```python
from build123d import *

# Parameters (mm, degrees)
SKETCH1_W           = 61
SKETCH1_H           = 36
SKETCH1_R           = 2.5
BOSS_EXTRUDE1_DEPTH = 5
BOSS_EXTRUDE3_START = -18
BOSS_EXTRUDE3_DEPTH = 6
BOSS_EXTRUDE2_DEPTH = 12
FILLET1_R           = 1.5
FILLET2_R           = 1.5
FILLET3_R           = 1.5
FILLET4_R           = 1.5
SKETCH5_W           = 61
SKETCH5_H           = 36
SKETCH5_R           = 2.5
BOSS_EXTRUDE4_DEPTH = 5
FILLET5_R           = 1.5
FILLET6_R           = 1.5
FILLET7_R           = 1.5


with BuildPart() as part:
    # Sketch1 → Boss-Extrude1 (new body)
    with BuildSketch(Plane(origin=(0, 0, 0), x_dir=(1, 0, 0), z_dir=(0, 1, 0))):
        Rectangle(SKETCH1_W, SKETCH1_H)
        with Locations(Location((-25.5, 13.49396263, 0), (0, 0, 270))):
            Circle(SKETCH1_R, mode=Mode.SUBTRACT)
        with Locations(Location((25.5, 13.49396263, 0), (0, 0, 270))):
            Circle(SKETCH1_R, mode=Mode.SUBTRACT)
        with Locations(Location((25.5, -13, 0), (0, 0, 270))):
            Circle(SKETCH1_R, mode=Mode.SUBTRACT)
        with Locations(Location((-25.5, -13, 0), (0, 0, 270))):
            Circle(SKETCH1_R, mode=Mode.SUBTRACT)
    extrude(amount=BOSS_EXTRUDE1_DEPTH)

    # Sketch4 → Boss-Extrude3 (add, symmetric)
    with BuildSketch(Plane.XY.offset(18).offset(BOSS_EXTRUDE3_START)):
        Polygon((19.75, 5), (-17.25, 35), (-27.25, 35), (9.75, 5), align=None)
    extrude(amount=BOSS_EXTRUDE3_DEPTH, both=True)

    # Sketch3 → Boss-Extrude2 (add)
    with BuildSketch(Plane.XY.offset(18)):
        Polygon((-19.75, 5), (11.5, 35), (21.5, 35), (-9.75, 5), align=None)
    boss_extrude2 = extrude(amount=-BOSS_EXTRUDE2_DEPTH)

    # Mirror1: Boss-Extrude2 across plane
    add(boss_extrude2.mirror(Plane.XY))

    # Fillet1
    fillet1_edges = [part.edges().sort_by_distance(p)[0] for p in [
        (-9.75, 5, 12),
    ]]
    fillet(fillet1_edges, radius=FILLET1_R)

    # Fillet2
    fillet2_edges = [part.edges().sort_by_distance(p)[0] for p in [
        (-9.75, 5, -12),
    ]]
    fillet(fillet2_edges, radius=FILLET2_R)

    # Fillet3
    fillet3_edges = [part.edges().sort_by_distance(p)[0] for p in [
        (9.75, 5, 0),
    ]]
    fillet(fillet3_edges, radius=FILLET3_R)

    # Fillet4
    fillet4_edges = [part.edges().sort_by_distance(p)[0] for p in [
        (19.75, 5, 0),
        (-19.75, 5, 12),
        (-19.75, 5, -12),
    ]]
    fillet(fillet4_edges, radius=FILLET4_R)

    # Sketch5 → Boss-Extrude4 (add)
    with BuildSketch(Plane(origin=(0, 35, 0), x_dir=(1, 0, 0), z_dir=(0, 1, 0))):
        Rectangle(SKETCH5_W, SKETCH5_H)
        with Locations(Location((-25.5, -13, 0), (0, 0, 270))):
            Circle(SKETCH5_R, mode=Mode.SUBTRACT)
        with Locations(Location((-25.5, 13.49396263, 0), (0, 0, 270))):
            Circle(SKETCH5_R, mode=Mode.SUBTRACT)
        with Locations(Location((25.5, 13.49396263, 0), (0, 0, 270))):
            Circle(SKETCH5_R, mode=Mode.SUBTRACT)
        with Locations(Location((25.5, -13, 0), (0, 0, 270))):
            Circle(SKETCH5_R, mode=Mode.SUBTRACT)
    extrude(amount=BOSS_EXTRUDE4_DEPTH)

    # Fillet5
    fillet5_edges = [part.edges().sort_by_distance(p)[0] for p in [
        (11.5, 35, 12),
    ]]
    fillet(fillet5_edges, radius=FILLET5_R)

    # Fillet6
    fillet6_edges = [part.edges().sort_by_distance(p)[0] for p in [
        (11.5, 35, -12),
    ]]
    fillet(fillet6_edges, radius=FILLET6_R)

    # Fillet7
    fillet7_edges = [part.edges().sort_by_distance(p)[0] for p in [
        (-17.25, 35, 0),
    ]]
    fillet(fillet7_edges, radius=FILLET7_R)


solid = part.part
```
Check sheet for the modelled part. Datum: model origin and axes. Units: mm. A direction names the side the tool comes from. Round coordinates to 2 decimals unless told otherwise and drop trailing zeros. Loops run counter-clockwise (first coordinate to the right, second up) from the corner with the lowest first, then second, coordinate; pieces in that order, holes last. Notation, with made-up numbers: (68.5, 20.25) - (81.5, 20.25) arc R23 cw to (81.5, 45.25) - close; hole circle Ø3 at (39, 66). An arc over 180 degrees is marked (long way). Answer as a JSON object with one key per item and string values. Group by question number.
Q1. Sectioned sample at A-A, the plane x = 25.5. Enter the section's corners in (y, z), plus the area to 3 significant figures.
Q2. Set-up check for faces 4 (the face through (-23.39, 2.46, -12.15)), 5 (the face through (-15, 28, -6)), 6 (the face through (0, 5, 0)), 7 (the face through (10, 28, 6)), 8 (the face through (-8, 10, -6)): record each of +Z, -Z, +X, -X, +Y, -Y from which the full face is reachable in a straight line by a thin tool's end or side.
Q3. Sectioned sample at C-C, the plane y = 30. Enter the section's corners in (x, z), plus the area to 3 significant figures.
Q4. Sectioned sample at B-B, the plane z = 13. Count the separate pieces of the cut face and the enclosed holes in it, plus the area to 3 significant figures.
Q5. Mould release check, pull along Z, two halves, no side actions. Record for faces 1 (the face through (28, 2, 13)), 2 (the face through (7, 10, -6)), 3 (the face through (30.5, 2, 0)): released by +Z, released by -Z, zero draft, split by the parting line, or undercut.
Q6. Scan lines: line 1 along X through (y, z) = (39, 13); line 2 along Z through (x, y) = (-24.5, 2); line 3 along Z through (x, y) = (-9, 6). Record each from-to range of solid material in increasing order. Write a range as [from, to].
Q7. Sectioned sample at D-D, the plane x = 2. Enter the section's corners in (y, z).
Q8. Gauge pin test, flat ends, axial feed: P1, Ø2, axis at x = -24.5, y = 6.5, coming from the +Z side; P2, Ø4, axis at y = 32.5, z = -5.5, coming from the +X side; P3, Ø5, axis at x = -18.5, y = 29, coming from the +Z side; P4, Ø5, axis at x = -15.5, y = 30, coming from the -Z side. Record the tip position at first contact, or that the pin passes through.
Solution:
{
 "1": {"outline": "(0, -18) - (5, -18) - (5, -15.99) - (0, -15.99) - close; (0, -10.99) - (5, -10.99) - (5, 10.5) - (0, 10.5) - close; (0, 15.5) - (5, 15.5) - (5, 18) - (0, 18) - close; (35, -18) - (40, -18) - (40, -15.99) - (35, -15.99) - close; (35, -10.99) - (40, -10.99) - (40, 10.5) - (35, 10.5) - close; (35, 15.5) - (40, 15.5) - (40, 18) - (35, 18) - close", "area": "260 mm²"},
 "2": {"face 4": "+Y, -Y", "face 5": "-Z, -X", "face 6": "none", "face 7": "+X", "face 8": "-X"},
 "3": {"outline": "(-21.08, -6) - (-11.08, -6) - (-11.08, 6) - (-21.08, 6) - close; (6.29, -18) - (16.29, -18) - (16.29, -6) - (6.29, -6) - close; (6.29, 6) - (16.29, 6) - (16.29, 18) - (6.29, 18) - close", "area": "360 mm²"},
 "4": {"separate pieces": "5", "enclosed holes": "0", "area": "816 mm²"},
 "5": {"face 1": "undercut", "face 2": "released by -Z", "face 3": "zero draft"},
 "6": {"line 1": "x = [-30.5, -28], [-23, 23], [28, 30.5]", "line 2": "z = [-18, -15.79], [-11.2, 10.71], [15.29, 18]", "line 3": "z = [-18, -6], [6, 18]"},
 "7": {"outline": "(0, -18) - (5, -18) - (5, 18) - (0, 18) - close; (11.28, -6) - (16.28, -6) - (16.28, -18) - (25.88, -18) - (25.88, -6) - (19.39, -6) - (19.39, 6) - (25.88, 6) - (25.88, 18) - (16.28, 18) - (16.28, 6) - (11.28, 6) - close; (35, -18) - (40, -18) - (40, 18) - (35, 18) - close"},
 "8": {"P1": "passes through", "P2": "stops at x = 20.91", "P3": "stops at z = 6", "P4": "stops at z = -6"}
}
